```python
from build123d import *

# Parameters (mm, degrees)
SKETCH4_R           = 10
BOSS_EXTRUDE2_DEPTH = 6
CUT_EXTRUDE2_DEPTH  = 30


with BuildPart() as part:
    # Sketch1 → Revolve1 (revolve)
    with BuildSketch(Plane.XY, mode=Mode.PRIVATE) as revolve1_sk:
        with BuildLine():
            Line((20.9, 0), (23.871591838, 0))
            Line((23.871591838, 0), (23.871591838, 4))
            Line((23.871591838, 4), (22.9, 4.236662843))
            Line((22.9, 4.236662843), (22.9, 36.5))
            ThreePointArc((22.9, 36.5), (21.874873734, 38.974873734), (19.4, 40))
            Line((19.4, 40), (0, 40))
            Line((0, 40), (0, 38))
            Line((0, 38), (18.9, 38))
            ThreePointArc((18.9, 38), (20.314213562, 37.414213562), (20.9, 36))
            Line((20.9, 36), (20.9, 13.908178136))
            Line((20.9, 13.908178136), (0, 13.908178136))
            Line((0, 13.908178136), (0, 11.908178136))
            Line((0, 11.908178136), (20.9, 11.908178136))
            Line((20.9, 11.908178136), (20.9, 0))
        make_face()
    revolve(revolve1_sk.sketch.rotate(Axis((0, -0.724089275, 0), (0, 1, 0)), 90), axis=Axis((0, -0.724089275, 0), (0, 1, 0)))

    # Sketch4 → Boss-Extrude2 (add)
    with BuildSketch(Plane.XY.offset(22.9)):
        with Locations((1.144629865, 24.5)):
            Circle(SKETCH4_R)
    extrude(amount=-BOSS_EXTRUDE2_DEPTH)

    # Sketch9 → Cut-Extrude2 (cut)
    with BuildSketch(Plane(origin=(0, 40, 0), x_dir=(1, 0, 0), z_dir=(0, 1, 0))):
        with BuildLine():
            Line((-20.5, 0), (20.5, 0))
            ThreePointArc((20.5, 0), (0, 20.5), (-20.5, 0))
        make_face()
    extrude(amount=-CUT_EXTRUDE2_DEPTH, mode=Mode.SUBTRACT)


solid = part.part
```
Model file for the job. Use its own axes, mm. A direction names the side the tool comes from. Coordinates: 2 decimals unless noted, no trailing zeros. Loops run counter-clockwise (first coordinate to the right, second up) from the corner with the lowest first, then second, coordinate; pieces in that order, holes last. Notation, with made-up numbers: (55, 74) - (112, 74) arc R18 cw to (112, 79) - close; hole circle Ø8 at (-23, 83). An arc over 180 degrees is marked (long way). Answer as a JSON object with one key per item and string values. Group by question number.
(1) Two-plate mould, pull along X, no slides. Class faces 4 (the face through (0, 11.908, 9)), 5 (the face through (-23.67, 2.03, 3.11)), 6 (the face through (0, 40, 8)): released by +X, released by -X, zero draft, split by the parting line, or undercut.
(2) Flat gauge pins, fed straight in: pin 1 (12 mm diameter, centred on x = 12, y = 34.5, fed in from -Z); pin 2 (3 mm diameter, centred on x = 9, y = 38, fed in from -Z); pin 3 (6 mm diameter, centred on x = 14.5, y = 22.5, fed in from -Z); pin 4 (5 mm diameter, centred on x = -14, z = -18, fed in from -Y). Where does each tip first touch, or does it go through?
(3) Probe line 1 along Y through (x, z) = (-11, 5.5); line 2 along X through (y, z) = (9, 0); line 3 along X through (y, z) = (38, -8.5). List the from-to ranges inside material, lowest first.
(4) Cut at B-B (y = 24.5). Give the cut face in (x, z).
(5) Tool access for faces 1 (the face through (-6.278, 5.871, -19.935)), 2 (the face through (0, 13, 0)), 3 (the face through (-8.853, 24.704, 22.22)): list every direction of +Z, -Z, +X, -X, +Y, -Y with a clear straight run to the whole face (end or side of a thin tool).
(6) Cut at C-C (y = 9). Give the cut face in (x, z).
(7) Cut at A-A (y = 31). Give the cut face in (x, z), then the cut area to 3 significant figures.
Geometry says:
{
 "1": {"face 4": "undercut", "face 5": "split by the parting line", "face 6": "zero draft"},
 "2": {"pin 1": "stops at z = -22.1", "pin 2": "stops at z = -21.48", "pin 3": "stops at z = -19.8", "pin 4": "stops at y = 0"},
 "3": {"line 1": "y = 11.91 to 13.91, 38 to 40", "line 2": "x = -22.9 to -20.9, 20.9 to 22.9", "line 3": "x = -20.9 to -18.65, 18.65 to 20.9"},
 "4": {"outline": "(-8.86, 21.12) arc R22.9 ccw (long way) to (11.14, 20.01) - (11.14, 22.9) - (-8.86, 22.9) - close; hole (-8.86, 16.9) - (-8.86, 18.93) arc R20.9 ccw (long way) to (11.14, 17.68) - (11.14, 16.9) - close"},
 "5": {"face 1": "-Y", "face 2": "+Y, -Y", "face 3": "+Z, -X"},
 "6": {"outline": "circle Ø45.8 at (0, 0); hole circle Ø41.8 at (0, 0)"},
 "7": {"outline": "(-6.45, 21.97) arc R22.9 ccw (long way) to (8.74, 21.16) - (8.74, 22.9) - (-6.45, 22.9) - close; hole (-6.45, 16.9) - (-6.45, 19.88) arc R20.9 ccw (long way) to (8.74, 18.98) - (8.74, 16.9) - close", "area": "335 mm^2"}
}
